```python
from build123d import *

# Parameters (mm, degrees)
F0_R     = 11.2
F1_DEPTH = 7


with BuildPart() as f1:
    # F0 (on Top) → F1 (new body)
    with BuildSketch(Plane.XY):
        with BuildLine():
            ThreePointArc((-5.3140176456, 19.2319211805), (1.6632130225, 18.2202199581), (8.1659804164, 20.9440597808))
            ThreePointArc((8.1659804164, 20.9440597808), (11.8749935052, 25.5509452113), (13.2, 31.3150174916))
            ThreePointArc((13.2, 31.3150174916), (-7.2143941907, 42.3690898842), (-5.3140176456, 19.2319211805))
        make_face()
        with Locations((0, 31.3150174916)):
            Circle(F0_R, mode=Mode.SUBTRACT)
        with BuildLine():
            ThreePointArc((-13.9196006677, -15.6575087458), (-13.939296065, -14.9366963), (-13.9983234831, -14.2180348675))
            ThreePointArc((-13.9983234831, -14.2180348675), (-16.6107798575, -7.6697252497), (-22.2210780368, -3.400083403))
            ThreePointArc((-22.2210780368, -3.400083403), (-38.0489304442, -23.0595186509), (-13.9196006677, -15.6575087458))
        make_face()
        with Locations((-27.1196006677, -15.6575087458)):
            Circle(F0_R, mode=Mode.SUBTRACT)
        with BuildLine():
            ThreePointArc((0.6623638429, -13.183371122), (9.565124221, -9.09661468), (13.2, 0))
            ThreePointArc((13.2, 0), (13.0393347088, 2.0532292498), (12.5612499466, 4.0564762761))
            ThreePointArc((12.5612499466, 4.0564762761), (11.7880076827, 5.5940019812), (11.0859523777, 7.1653094754))
            ThreePointArc((11.0859523777, 7.1653094754), (1.0616824394, 13.157234907), (-9.7936364782, 8.850123419))
            ThreePointArc((-9.7936364782, 8.850123419), (-10.7385516659, 7.4117131226), (-11.7483162206, 6.0180616465))
            ThreePointArc((-11.7483162206, 6.0180616465), (-11.9253408927, -5.6591734902), (-2.7676134684, -12.9065996951))
            ThreePointArc((-2.7676134684, -12.9065996951), (-1.0494560168, -13.0057151038), (0.6623638429, -13.183371122))
        make_face()
        Circle(F0_R, mode=Mode.SUBTRACT)
        with BuildLine():
            ThreePointArc((12.5612499466, 4.0564762761), (13.0393347088, 2.0532292498), (13.2, 0))
            ThreePointArc((13.2, 0), (9.565124221, -9.09661468), (0.6623638429, -13.183371122))
            ThreePointArc((0.6623638429, -13.183371122), (7.5647950779, -14.7307879991), (14.0550976203, -17.5439763778))
            ThreePointArc((14.0550976203, -17.5439763778), (14.947566835, -10.5504947085), (19.3123411287, -5.013886313))
            ThreePointArc((19.3123411287, -5.013886313), (15.5937950375, -0.7340010586), (12.5612499466, 4.0564762761))
        make_face()
        with BuildLine():
            ThreePointArc((40.3196006677, -15.6575087458), (33.0855110796, -3.8826239074), (19.3123411287, -5.013886313))
            ThreePointArc((19.3123411287, -5.013886313), (14.947566835, -10.5504947085), (14.0550976203, -17.5439763778))
            ThreePointArc((14.0550976203, -17.5439763778), (28.0652643963, -28.8235909312), (40.3196006677, -15.6575087458))
        make_face()
        with Locations((27.1196006677, -15.6575087458)):
            Circle(F0_R, mode=Mode.SUBTRACT)
        with BuildLine():
            ThreePointArc((-9.7936364782, 8.850123419), (1.0616824394, 13.157234907), (11.0859523777, 7.1653094754))
            ThreePointArc((11.0859523777, 7.1653094754), (8.9748390861, 13.9166987115), (8.1659804164, 20.9440597808))
            ThreePointArc((8.1659804164, 20.9440597808), (1.6632130225, 18.2202199581), (-5.3140176456, 19.2319211805))
            ThreePointArc((-5.3140176456, 19.2319211805), (-7.1612339556, 13.8716231732), (-9.7936364782, 8.850123419))
        make_face()
        with BuildLine():
            ThreePointArc((-13.9983234831, -14.2180348675), (-8.432561082, -13.1376221146), (-2.7676134684, -12.9065996951))
            ThreePointArc((-2.7676134684, -12.9065996951), (-11.9253408927, -5.6591734902), (-11.7483162206, 6.0180616465))
            ThreePointArc((-11.7483162206, 6.0180616465), (-16.539634164, 0.8140892877), (-22.2210780368, -3.400083403))
            ThreePointArc((-22.2210780368, -3.400083403), (-16.6107798575, -7.6697252497), (-13.9983234831, -14.2180348675))
        make_face()
    extrude(amount=F1_DEPTH)


solid = f1.part
```
Geometry: final body of the model. Coordinates: model frame, mm. Round coordinates to 2 decimals unless told otherwise and drop trailing zeros. Order: outer loops, then holes, each group sorted by start corner. A loop starts at its lowest first (then second) coordinate and runs counter-clockwise, first axis right, second up. Notation, with made-up numbers: (-6.5, 4.25) - (43.5, 4.25) arc R9 cw to (43.5, 20.25) - close; hole circle Ø9 at (76.25, 9). An arc over 180 degrees is marked (long way). Use CSV: the item, a comma, the result in double quotes. Start each with the question number.
Q1. First-contact query: pin 1 (3 mm diameter, centred on x = -32, z = 1.5, fed in from +Y); pin 2 (1 mm diameter, centred on x = 5, z = 4.5, fed in from -Y); pin 3 (1 mm diameter, centred on x = -18.5, z = 2, fed in from +Y). Flat tips, straight axial feed; report the tip coordinate or a pass-through.
Q2. Mould query, pull axis X, two halves, no side actions, for faces 1 (the face through (3, -11, 0)), 2 (the face through (-11.19, 0.49, 3.45)). Classes: +X half, -X half, draft (parallel to the pull), parting line (faces both ways), or undercut.
Q3. Material intervals for line 1 along Y through (x, z) = (8, 6.5); line 2 along Y through (x, z) = (-2.5, 0.75); line 3 along Y through (x, z) = (-9, 6.75), sorted ascending. Write a range as from..to.
Q4. Section query A-A (z = 2). Return loops of the section in (x, y).
Q5. Section query D-D (y = -19). Return loops of the section in (x, z), and give its area (3 significant figures).
Q6. Section query C-C (y = 24). Return loops of the section in (x, z), and give its area (3 significant figures).
Q7. Section query B-B (x = 35). Return loops of the section in (y, z), and give its area (3 significant figures).
Result set:
1,pin 1,"stops at y = -2.9"
1,pin 2,"stops at y = -14.12"
1,pin 3,"stops at y = -0.43"
2,face 1,"draft"
2,face 2,"undercut"
3,line 1,"y = -14.88..-7.84, 7.84..23.48, 39.15..41.81"
3,line 2,"y = -12.92..-10.92, 10.92..20.4, 42.23..44.28"
3,line 3,"y = -13.21..-6.67, 6.67..10.18, 21.66..24.65, 37.98..40.97"
4,outline,"(-22.22, -3.4) arc R13.2 ccw (long way) to (-14, -14.22) arc R37.59 cw to (14.06, -17.54) arc R13.2 ccw (long way) to (19.31, -5.01) arc R37.59 cw to (8.17, 20.94) arc R13.2 ccw (long way) to (-5.31, 19.23) arc R37.59 cw to start; hole circle Ø22.4 at (-27.12, -15.66); hole circle Ø22.4 at (0, 0); hole circle Ø22.4 at (0, 31.32); hole circle Ø22.4 at (27.12, -15.66)"
5,outline,"(-39.89, 0) - (-37.81, 0) - (-37.81, 7) - (-39.89, 7) - close; (-16.43, 0) - (-14.35, 0) - (-14.35, 7) - (-16.43, 7) - close; (14.35, 0) - (16.43, 0) - (16.43, 7) - (14.35, 7) - close; (37.81, 0) - (39.89, 0) - (39.89, 7) - (37.81, 7) - close"
5,area,"58.2 mm2"
6,outline,"(-10.99, 0) - (-8.48, 0) - (-8.48, 7) - (-10.99, 7) - close; (8.48, 0) - (10.99, 0) - (10.99, 7) - (8.48, 7) - close"
6,area,"35.1 mm2"
7,outline,"(-26.25, 0) - (-23.62, 0) - (-23.62, 7) - (-26.25, 7) - close; (-7.7, 0) - (-5.07, 0) - (-5.07, 7) - (-7.7, 7) - close"
7,area,"36.8 mm2"
